from build123d import *

# Parameters (mm, degrees)
CROQUIS1_W              = 34
CROQUIS1_H              = 30
SALIENTE_EXTRUIR1_DEPTH = 4
CROQUIS2_W              = 6
CROQUIS2_H              = 4
SALIENTE_EXTRUIR2_DEPTH = 4
CORTAR_EXTRUIR1_DEPTH   = 5
CROQUIS4_W              = 6
CROQUIS4_H              = 2
SALIENTE_EXTRUIR3_DEPTH = 4
CROQUIS5_R              = 1.5
CORTAR_EXTRUIR2_DEPTH   = 5
CORTAR_EXTRUIR4_DEPTH   = 5
CORTAR_EXTRUIR6_DEPTH   = 5


with BuildPart() as part:
    # Croquis1 → Saliente-Extruir1 (new body)
    with BuildSketch(Plane(origin=(0, 0, 0), x_dir=(0, -1, 0), z_dir=(1, 0, 0))):
        Rectangle(CROQUIS1_W, CROQUIS1_H)
    extrude(amount=SALIENTE_EXTRUIR1_DEPTH)

    # Croquis2 → Saliente-Extruir2 (add, through all)
    with BuildSketch(Plane(origin=(4, 0, 0), x_dir=(0, 0, -1), z_dir=(1, 0, 0))):
        with Locations((-8, -19)):
            Rectangle(CROQUIS2_W, CROQUIS2_H)
        with Locations((8, -19)):
            Rectangle(CROQUIS2_W, CROQUIS2_H)
        with Locations((8, 19)):
            Rectangle(CROQUIS2_W, CROQUIS2_H)
        with Locations((-8, 19)):
            Rectangle(CROQUIS2_W, CROQUIS2_H)
    extrude(amount=-SALIENTE_EXTRUIR2_DEPTH)

    # Croquis3 → Cortar-Extruir1 (cut, through all)
    with BuildSketch(Plane(origin=(4, 0, 0), x_dir=(0, 0, -1), z_dir=(1, 0, 0))):
        Polygon((-1.55, 17), (-1.55, 14.95), (-2.8, 14.95), (-2.8, 12.05), (-1.55, 12.05), (-1.55, 10), (1.55, 10), (1.55, 12.05), (2.8, 12.05), (2.8, 14.95), (1.55, 14.95), (1.55, 17), align=None)
        Polygon((1.55, -12.05), (2.8, -12.05), (2.8, -14.95), (1.55, -14.95), (1.55, -17), (-1.55, -17), (-1.55, -14.95), (-2.8, -14.95), (-2.8, -12.05), (-1.55, -12.05), (-1.55, -10), (1.55, -10), align=None)
    extrude(amount=-CORTAR_EXTRUIR1_DEPTH, mode=Mode.SUBTRACT)

    # Croquis4 → Saliente-Extruir3 (add, through all)
    with BuildSketch(Plane(origin=(4, 0, 0), x_dir=(0, 0, -1), z_dir=(1, 0, 0))):
        with Locations((-8, -22)):
            Rectangle(CROQUIS4_W, CROQUIS4_H)
        with Locations((8, -22)):
            Rectangle(CROQUIS4_W, CROQUIS4_H)
    extrude(amount=-SALIENTE_EXTRUIR3_DEPTH)

    # Croquis5 → Cortar-Extruir2 (cut, through all)
    with BuildSketch(Plane(origin=(4, 0, 0), x_dir=(0, 0, -1), z_dir=(1, 0, 0))):
        with Locations((-12.060660172, -18.060660172)):
            Circle(CROQUIS5_R)
        with Locations((-3.939339828, -18.060660172)):
            Circle(CROQUIS5_R)
        with Locations((12.060660172, -18.060660172)):
            Circle(CROQUIS5_R)
        with Locations((3.939339828, -18.060660172)):
            Circle(CROQUIS5_R)
        with Locations((-12.060660172, 18.060660172)):
            Circle(CROQUIS5_R)
        with Locations((-3.939339828, 18.060660172)):
            Circle(CROQUIS5_R)
        with Locations((3.939339828, 18.060660172)):
            Circle(CROQUIS5_R)
        with Locations((12.060660172, 18.060660172)):
            Circle(CROQUIS5_R)
    extrude(amount=-CORTAR_EXTRUIR2_DEPTH, mode=Mode.SUBTRACT)

    # Croquis6 → Cortar-Extruir4 (cut, through all)
    with BuildSketch(Plane(origin=(4, 0, 0), x_dir=(0, 0, -1), z_dir=(1, 0, 0))):
        with BuildLine():
            ThreePointArc((0, -9.64272275), (-1.989339828, -11.060660172), (0, -12.478597594))
            ThreePointArc((0, -12.478597594), (1.989339828, -11.060660172), (0, -9.64272275))
        make_face()
        with BuildLine():
            ThreePointArc((0, 9.64272275), (-1.989339828, 11.060660172), (0, 12.478597594))
            ThreePointArc((0, 12.478597594), (1.989339828, 11.060660172), (0, 9.64272275))
        make_face()
    extrude(amount=-CORTAR_EXTRUIR4_DEPTH, mode=Mode.SUBTRACT)

    # Croquis7 → Cortar-Extruir6 (cut, through all)
    with BuildSketch(Plane(origin=(4, 0, 0), x_dir=(0, 0, -1), z_dir=(1, 0, 0))):
        with BuildLine():
            ThreePointArc((-0.290749307, -13.5), (-1.739339828, -11.610660172), (-3.187930349, -13.5))
            ThreePointArc((-3.187930349, -13.5), (-1.739339828, -15.389339828), (-0.290749307, -13.5))
        make_face()
        with BuildLine():
            ThreePointArc((0.290749307, -13.5), (1.739339828, -11.610660172), (3.187930349, -13.5))
            ThreePointArc((3.187930349, -13.5), (1.739339828, -15.389339828), (0.290749307, -13.5))
        make_face()
        with BuildLine():
            ThreePointArc((0.290749307, 13.5), (1.739339828, 11.610660172), (3.187930349, 13.5))
            ThreePointArc((3.187930349, 13.5), (1.739339828, 15.389339828), (0.290749307, 13.5))
        make_face()
        with BuildLine():
            ThreePointArc((-0.290749307, 13.5), (-1.739339828, 15.389339828), (-3.187930349, 13.5))
            ThreePointArc((-3.187930349, 13.5), (-1.739339828, 11.610660172), (-0.290749307, 13.5))
        make_face()
    extrude(amount=-CORTAR_EXTRUIR6_DEPTH, mode=Mode.SUBTRACT)


solid = part.part
Input: part model. Units: mm. Frame: model coordinates. A direction names the side the tool comes from. Round coordinates to 2 decimals unless told otherwise and drop trailing zeros. Order: outer loops, then holes, each group sorted by start corner. A loop starts at its lowest first (then second) coordinate and runs counter-clockwise, first axis right, second up. Notation, with made-up numbers: (21, 37.5) - (73, 37.5) arc R30 ccw to (73, 67.5) - close; hole circle Ø6 at (-37, 5). An arc over 180 degrees is marked (long way). Use a Markdown table: item, result.
1. Access query for faces 1 (the face through (2, -21, -5)), 2 (the face through (2.03, 12.24, -2.96)), 3 (the face through (2, 17, 2)). Directions: +Z, -Z, +X, -X, +Y, -Y. A direction counts if a zero-diameter tool reaches every point of the face in a straight line with its end or side. Return the directions, or none.
Evaluation:
| item | result |
|---|---|
| face 1 | +X, -X, -Y |
| face 2 | +X, -X |
| face 3 | +X, -X, +Y |
2. Section C-C on z = -11.75. Return the cut outline in (x, y), then the cut area to 3 significant figures.
Evaluation:
| item | result |
|---|---|
| outline | (0, -16.59) - (4, -16.59) - (4, 16.59) - (0, 16.59) - close |
| area | 133 mm^2 |
3. Section D-D on z = -4. Return the cut outline in (x, y), then the cut area to 3 significant figures.
Evaluation:
| item | result |
|---|---|
| outline | (0, -16.56) - (4, -16.56) - (4, 16.56) - (0, 16.56) - close |
| area | 132 mm^2 |
4. Mould query, pull axis Z, two halves, no side actions, for faces 4 (the face through (2, 20, -11)), 5 (the face through (2, -17, -14)), 6 (the face through (2.03, 10.04, -1.59)), 7 (the face through (2, 20, 11)). Classes: +Z half, -Z half, draft (parallel to the pull), parting line (faces both ways), or undercut.
Evaluation:
| item | result |
|---|---|
| face 4 | -Z half |
| face 5 | draft |
| face 6 | undercut |
| face 7 | +Z half |
5. Section B-B on y = 10.5. Return the cut outline in (x, z), then the cut area to 3 significant figures.
Evaluation:
| item | result |
|---|---|
| outline | (0, -15) - (4, -15) - (4, -1.88) - (0, -1.88) - close; (0, 1.88) - (4, 1.88) - (4, 15) - (0, 15) - close |
| area | 105 mm^2 |
6. First-contact query: pin 1 (1.5 mm diameter, centred on x = 2.5, z = -2.5, fed in from +Y); pin 2 (1.5 mm diameter, centred on x = 1.5, y = 19.5, fed in from +Z); pin 3 (0.9 mm diameter, centred on x = 1, y = 20, fed in from -Z). Flat tips, straight axial feed; report the tip coordinate or a pass-through.
Evaluation:
| item | result |
|---|---|
| pin 1 | y = 17 |
| pin 2 | z = 11 |
| pin 3 | z = -11 |
7. Section A-A on y = -16. Return the cut outline in (x, z).
Evaluation:
| item | result |
|---|---|
| outline | (0, -15) - (4, -15) - (4, -1.55) - (0, -1.55) - close; (0, 1.55) - (4, 1.55) - (4, 15) - (0, 15) - close |
8. Material intervals for probe 1 along Z at (x, y) = (2.75, 13); probe 2 along Z at (x, y) = (2.1, 15.5); probe 3 along Y at (x, z) = (3.5, -1.75), sorted ascending.
Evaluation:
| item | result |
|---|---|
| probe 1 | -15 to -3.24, 3.24 to 15 |
| probe 2 | -15 to -1.55, 1.55 to 15 |
| probe 3 | -17 to -15.39, -10.25 to 10.25, 15.39 to 17 |
